Read the model definition and answer for the solid it produces. Units are mm, in the model's axes. Face numbers are marked on the shaded views. Coordinates: 2 decimals unless noted, no trailing zeros. Write each loop counter-clockwise with the first axis right and the second up, starting at its lowest first coordinate (ties: lowest second). Pieces come first, ordered by that corner, then holes.
Item 1: Straight lines are drawn through the part: probe 1 along X at (y, z) = (2.5, 0); probe 2 along X at (y, z) = (-33, 0) (3 decimals); probe 3 along X at (y, z) = (-30.5, -111.5). For each, find the intervals that lie inside material, in ascending order.
Item 2: Section A-A (y = -21.5) is taken. Give the vertices of the cut face in (x, z) (3 decimals).
Item 3: Each of these flat-tipped pins is pushed along its axis until it touches: P1, Ø1.5, axis at x = 140, y = -27, coming from the +Z side; P2, Ø1, axis at x = -24.5, y = -6.5, coming from the -Z side; P3, Ø1, axis at y = -2, z = 44.5, coming from the +X side. Where does it stop, or does it pass through?
Item 4: Determine the mould class of the marked faces 1 and 2 for opening direction X: released by +X, released by -X, zero draft, split by the parting line, or undercut.
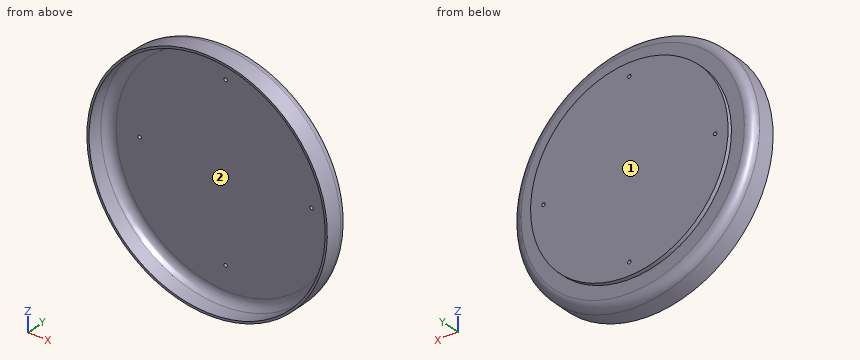
from build123d import *

# Parameters (mm, degrees)
SKETCH1_R           = 146.05
BOSS_EXTRUDE1_DEPTH = 6.35
SKETCH2_R           = 177.8
BOSS_EXTRUDE2_DEPTH = 38.1
SKETCH3_R           = 174.625
CUT_EXTRUDE2_DEPTH  = 34.925
FILLET2_R           = 12.7
FILLET3_R           = 12.7
SKETCH4_R           = 2.54
CUT_EXTRUDE3_DEPTH  = 9.525


with BuildPart() as part:
    # Sketch1 → Boss-Extrude1 (new body)
    with BuildSketch(Plane(origin=(0, 0, 0), x_dir=(1, 0, 0), z_dir=(0, 1, 0))):
        with Locations(Location((0, 0, 0), (0, 0, 270))):
            Circle(SKETCH1_R)
    extrude(amount=BOSS_EXTRUDE1_DEPTH)

    # Sketch2 → Boss-Extrude2 (add)
    with BuildSketch(Plane.XZ):
        with Locations(Location((0, 0, 0), (0, 0, 90))):
            Circle(SKETCH2_R)
    extrude(amount=BOSS_EXTRUDE2_DEPTH)

    # Sketch3 → Cut-Extrude2 (cut)
    with BuildSketch(Plane.XZ.offset(38.1)):
        with Locations(Location((0, 0, 0), (0, 0, 270))):
            Circle(SKETCH3_R)
    extrude(amount=-CUT_EXTRUDE2_DEPTH, mode=Mode.SUBTRACT)

    # Fillet2
    fillet2_edges = [part.edges().sort_by_distance(p)[0] for p in [
        (0, -3.175, 174.625),
    ]]
    fillet(fillet2_edges, radius=FILLET2_R)

    # Fillet3
    fillet3_edges = [part.edges().sort_by_distance(p)[0] for p in [
        (0, 0, -177.8),
    ]]
    fillet(fillet3_edges, radius=FILLET3_R)

    # Sketch4 → Cut-Extrude3 (cut)
    with BuildSketch(Plane(origin=(0, 6.35, 0), x_dir=(1, 0, 0), z_dir=(0, 1, 0))):
        with Locations(Location((0, 127, 0), (0, 0, 270))):
            Circle(SKETCH4_R)
        with Locations(Location((127, 0, 0), (0, 0, 270))):
            Circle(SKETCH4_R)
        with Locations(Location((-127, 0, 0), (0, 0, 270))):
            Circle(SKETCH4_R)
        with Locations(Location((0, -127, 0), (0, 0, 270))):
            Circle(SKETCH4_R)
    extrude(amount=-CUT_EXTRUDE3_DEPTH, mode=Mode.SUBTRACT)


solid = part.part
Established:
1. probe 1: x = -146.05 to -129.54, -124.46 to 124.46, 129.54 to 146.05
1. probe 2: x = -177.8 to -174.625, 174.625 to 177.8
1. probe 3: x = -138.49 to -134.39, 134.39 to 138.49
2. outline: circle Ø355.6 at (0, 0); hole circle Ø349.25 at (0, 0)
3. P1: stops at z = 110.55
3. P2: stops at z = -174.75
3. P3: stops at x = 166.85
4. face 1: zero draft
4. face 2: undercut
